Check sheet for the modelled part. Datum: model origin and axes. Units: mm. Face numbers are marked on the shaded views. A direction names the side the tool comes from. Coordinates: 2 decimals unless noted, no trailing zeros. Loops run counter-clockwise (first coordinate to the right, second up) from the corner with the lowest first, then second, coordinate; pieces in that order, holes last. Notation, with made-up numbers: M 64,85.5 L 91,85.5 A17 ccw 91,106.5 Z; hole C 44.25,88 d6. An arc over 180 degrees is marked long. Return JSON: item names as keys, results as strings.
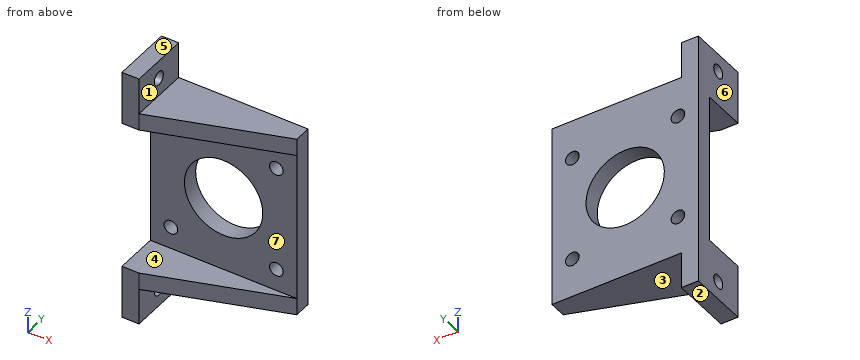
from build123d import *

# Parameters (mm, degrees)
SKETCH1_W           = 5
SKETCH1_H           = 5
SKETCH1_W_2         = 38
BOSS_EXTRUDE1_DEPTH = 44
SKETCH2_R           = 11.5
SKETCH2_R_2         = 2
CUT_EXTRUDE1_DEPTH  = 62.725197448
SKETCH1_3_W         = 38
SKETCH1_3_H         = 5
SKETCH1_3_W_2       = 5
SKETCH1_3_H_2       = 12.666
BOSS_EXTRUDE2_DEPTH = 5
BOSS_EXTRUDE3_START = -44
SKETCH1_4_W         = 5
SKETCH1_4_H         = 5
SKETCH1_4_H_2       = 12.666
SKETCH1_4_W_2       = 38
BOSS_EXTRUDE3_DEPTH = 5
SKETCH3_W           = 10.666
SKETCH3_H           = 17.666
SKETCH3_R           = 2
BOSS_EXTRUDE4_DEPTH = 5


with BuildPart() as part:
    # Sketch1 → Boss-Extrude1 (new body)
    with BuildSketch(Plane.XY):
        with Locations((2.5, 2.5)):
            Rectangle(SKETCH1_W, SKETCH1_H)
        with Locations((24, 2.5)):
            Rectangle(SKETCH1_W_2, SKETCH1_H)
    extrude(amount=-BOSS_EXTRUDE1_DEPTH)

    # Sketch2 → Cut-Extrude1 (cut, through all)
    with BuildSketch(Plane(origin=(0, 5, 0), x_dir=(1, 0, 0), z_dir=(0, 1, 0))):
        with Locations(Location((21.5, 22, 0), (0, 0, 270))):
            Circle(SKETCH2_R)
        with Locations(Location((37, 37.5, 0), (0, 0, 270))):
            Circle(SKETCH2_R_2)
        with Locations(Location((6, 37.5, 0), (0, 0, 270))):
            Circle(SKETCH2_R_2)
        with Locations(Location((6, 6.5, 0), (0, 0, 270))):
            Circle(SKETCH2_R_2)
        with Locations(Location((37, 6.5, 0), (0, 0, 270))):
            Circle(SKETCH2_R_2)
    extrude(amount=-CUT_EXTRUDE1_DEPTH, mode=Mode.SUBTRACT)

    # Sketch1<3> → Boss-Extrude2 (add)
    with BuildSketch(Plane.XY):
        Polygon((5, 0), (5, -12.666), (43, 0), align=None)
        with Locations((24, 2.5)):
            Rectangle(SKETCH1_3_W, SKETCH1_3_H)
        with Locations((2.5, 2.5)):
            Rectangle(SKETCH1_3_W_2, SKETCH1_3_H)
        with Locations((2.5, -6.333)):
            Rectangle(SKETCH1_3_W_2, SKETCH1_3_H_2)
    extrude(amount=BOSS_EXTRUDE2_DEPTH)

    # Sketch1<4> → Boss-Extrude3 (add)
    with BuildSketch(Plane.XY.offset(BOSS_EXTRUDE3_START)):
        with Locations((2.5, 2.5)):
            Rectangle(SKETCH1_4_W, SKETCH1_4_H)
        with Locations((2.5, -6.333)):
            Rectangle(SKETCH1_4_W, SKETCH1_4_H_2)
        Polygon((5, 0), (5, -12.666), (43, 0), align=None)
        with Locations((24, 2.5)):
            Rectangle(SKETCH1_4_W_2, SKETCH1_4_H)
    extrude(amount=-BOSS_EXTRUDE3_DEPTH)

    # Sketch3 → Boss-Extrude4 (add)
    # profile 1 of 2: a face of its own
    with BuildSketch(Plane.ZY):
        with Locations((10.333, -3.833)):
            Rectangle(SKETCH3_W, SKETCH3_H)
        with Locations((10.333, -3.833)):
            Circle(SKETCH3_R, mode=Mode.SUBTRACT)
    # profile 2 of 2: a face of its own
    with BuildSketch(Plane.ZY):
        with Locations((-54.333, -3.833)):
            Rectangle(SKETCH3_W, SKETCH3_H)
        with Locations(Location((-54.333, -3.833, 0), (0, 0, 180))):
            Circle(SKETCH3_R, mode=Mode.SUBTRACT)
    extrude(amount=-BOSS_EXTRUDE4_DEPTH)


solid = part.part
1) Scan lines: line 1 along X through (y, z) = (3.9, -37.5); line 2 along Z through (x, y) = (8, -9); line 3 along X through (y, z) = (0.75, 10). Record each from-to range of solid material in increasing order. Write a range as [from, to].
Answers:
{"line 1": "[0, 4], [8, 35], [39, 43]", "line 2": "[-49, -44], [0, 5]", "line 3": "[0, 5]"}
2) Section check B-B on x = 6. Record the cut outline in (y, z).
Answers:
{"outline": "M -12.33,-49 L 5,-49 L 5,-39.5 L 0,-39.5 L 0,-44 L -12.33,-44 Z; M -12.33,0 L 0,0 L 0,-4.5 L 5,-4.5 L 5,5 L -12.33,5 Z; M 0,-35.5 L 5,-35.5 L 5,-8.5 L 0,-8.5 Z"}
3) Go/stop test with flat-tipped pins: pin 1 Ø3 at (y, z) = (-4, 9.5) entering from +X; pin 2 Ø10 at (x, y) = (16.5, -7) entering from -Z; pin 3 Ø1.5 at (x, y) = (9.5, 1.5) entering from +Z. Record where each tip stops, or that it passes through.
Answers:
{"pin 1": "x = 5", "pin 2": "z = -49", "pin 3": "z = 5"}
4) Section check A-A on z = -37.5. Record the cut outline in (x, y), then the cut area to 3 significant figures.
Answers:
{"outline": "M 0,0 L 4,0 L 4,5 L 0,5 Z; M 8,0 L 35,0 L 35,5 L 8,5 Z; M 39,0 L 43,0 L 43,5 L 39,5 Z", "area": "175 mm²"}
5) Section check D-D on y = 1.25. Record the cut outline in (x, z), then the cut area to 3 significant figures.
Answers:
{"outline": "M 0,-59.67 L 5,-59.67 L 5,-49 L 43,-49 L 43,5 L 5,5 L 5,15.67 L 0,15.67 Z; hole C 6,-37.5 d4; hole C 6,-6.5 d4; hole C 21.5,-22 d23; hole C 37,-37.5 d4; hole C 37,-6.5 d4", "area": "1,960 mm²"}
6) Section check C-C on z = -22. Record the cut outline in (x, y), then the cut area to 3 significant figures.
Answers:
{"outline": "M 0,0 L 10,0 L 10,5 L 0,5 Z; M 33,0 L 43,0 L 43,5 L 33,5 Z", "area": "100 mm²"}
7) Draft check along Z on the marked faces 5, 6 and 7. Enter one of: +Z half, -Z half, draft (parallel to the pull), parting line (faces both ways), or undercut.
Answers:
{"face 5": "+Z half", "face 6": "draft", "face 7": "undercut"}
8) Set-up check for the marked faces 1, 2, 3 and 4: record each of +Z, -Z, +X, -X, +Y, -Y from which the full face is reachable in a straight line by a thin tool's end or side.
Answers:
{"face 1": "+Z, +X, +Y, -Y", "face 2": "-Z, +X, -X, +Y, -Y", "face 3": "-Z, +X, +Y, -Y", "face 4": "+X, -X, -Y"}
